Autodesk Inventor part; units mm, degrees
ref_plane "Work Plane1" through (0, 2.2914, -3.9688) normal (0, 0.8660254, 0.5) x (-1, 0, 0)
ref_plane "Work Plane2: Hex Center" through (-3.4449, 0, 0) normal (1, 0, 0) x (0, 0, -1)
ref_plane "YZ Plane" through (0, 0, 0) normal (1, 0, 0) x (0, 1, 0)
sketch "Sketch1: Hex" plane through (0, 0, 0) normal (1, 0, 0) x (0, 1, 0)
  line L0 (-2.2914, 3.9688) -> (2.2914, 3.9687)
  line L1 (2.2914, 3.9687) -> (4.5827, 0)
  line L2 (4.5827, 0) -> (2.2914, -3.9688)
  line L3 (2.2914, -3.9688) -> (-2.2914, -3.9688)
  line L4 (-2.2914, -3.9688) -> (-4.5827, 0)
  line L5 (-4.5827, 0) -> (-2.2914, 3.9688)
  circle A0 centre (0, 0) radius 0.87
  point P0 (0, 3.9687)
  point P1 (0, -3.9688)
  dimension "hex_angle" = 120
  dimension "hex_size" = 7.9375
  dimension "d1" = 1.7399
extrude "Ex: Hex" add sketch "Sketch1: Hex" against normal blind 6.8898 contours L0 L1 L2 L3 L4 L5 | A0
hole "Hole: Tap" [suppressed]
hole "Hole: Thread" at (0, 0, 0) direction (-1, 0, 0) diameter 3.683 depth 5.842
sketch "Sketch2: Top" plane through (-6.8898, 0, 0) normal (1, 0, 0) x (0, 1, 0)
  circle A0 centre (0, 0) radius 3.9687
  circle A1 centre (0, 0) radius 3.7147
  dimension "d4" = 7.9375
  dimension "d5" = 7.4295
extrude "Ex: Top" add sketch "Sketch2: Top" against normal blind 0.9843 contours A0 | A1
hole "Hole: Tubing" at (0, 0, 0) direction (-1, 0, 0) diameter 1.7399 end through all
chamfer "Chamfer1: Top (side)" distance 0.254 angle 45 1 edges at (-7.874, -3.9687, 0)
chamfer "Chamfer2: Top (hole)" distance 0.254 angle 45 1 edges at (-7.874, 0, 0.87)
sketch "Sketch3: Reference: Nut Chamfer" plane through (0, 0, 0) normal (1, 0, 0) x (0, 0, -1)
  circle A0 centre (0, 0) radius 3.9688
  line L0 (3.9688, 2.2914) -> (0, 4.5827)
ref_plane "Work Plane1" through (0, 2.2914, -3.9688) normal (0, 0.8660254, 0.5) x (-1, 0, 0)
sketch "Sketch4: Chamfer (nut)" plane through (0, 0, 0) normal (0, 0.8660254, 0.5) x (-1, 0, 0)
  line L0 (0, -3.9688) -> (0, -4.5827)
  line L1 (0, -4.5827) -> (0.3545, -4.5827)
  line L2 (0.3545, -4.5827) -> (0, -3.9688)
  line L3 (0, 3.9688) -> (0, -3.9688)
  line L4 (8.2677, 0) -> (-1.378, 0)
  line L5 (0, -4.5827) -> (6.8898, -4.5827)
  point P0 (0, 0)
  dimension "chamfer_angle" = 30
revolve "Revolution: Chamfer (nut)" cut sketch "Sketch4: Chamfer (nut)" angle 360 about axis through (-10, 0, 0) along (1, 0, 0)
ref_plane "Work Plane2: Hex Center" through (-3.4449, 0, 0) normal (1, 0, 0) x (0, 0, -1)
mirror "Mirror: Chamfer (nut)" about plane through (-3.4449, 0, 0) normal (1, 0, 0) of "Revolution: Chamfer (nut)"
properties part number "Nut for Precision Compression Fitting"
Geometry check sheet. Reference: the model listing, model coordinates, mm. Round coordinates to 2 decimals unless told otherwise and drop trailing zeros. Loops run counter-clockwise (first coordinate to the right, second up) from the corner with the lowest first, then second, coordinate; pieces in that order, holes last. Notation, with made-up numbers: M 84.25,68 L 135.25,68 A19 cw 135.25,73 Z; hole C 5.5,36 d11. An arc over 180 degrees is marked long. Return JSON: item names as keys, results as strings. Group by question number.
(1) Section check A-A, the plane x = -5.25. Enter the section's corners in (y, z), and give its area (3 significant figures).
(2) Section check B-B, the plane x = -6.25. Enter the section's corners in (y, z), and give its area (3 significant figures).
(3) Scan lines: line 1 along Z through (x, y) = (-2.5, 0); line 2 along Z through (x, y) = (-7.1, 0). Record each from-to range of solid material in increasing order. Write a range as [from, to].
(4) Mould release check, pull along Z, two halves, no side actions. Record for faces 1 (the face through (0, 1, -2)), 2 (the face through (-2.962, 1.634, -0.85)), 3 (the face through (-6.78, 2.09, 3.6)), 4 (the face through (-0.086, 4.118, 0.01)): pulls with the +Z half, pulls with the -Z half, needs draft (parallel to the pull), parting line crosses it, or undercut.
(5) Go/stop test with a flat-tipped pin: pin 1 (1.1 mm diameter, centred on y = 0, z = 0.5, fed in from +X). Record where the tip stops, or that it passes through.
Data:
{
 "1": {"outline": "M -4.58,0 L -2.29,-3.97 L 2.29,-3.97 L 4.58,0 L 2.29,3.97 L -2.29,3.97 Z; hole C 0,0 d3.68", "area": "43.9 mm²"},
 "2": {"outline": "M -4.58,0 L -2.29,-3.97 L 2.29,-3.97 L 4.58,0 L 2.29,3.97 L -2.29,3.97 Z; hole C 0,0 d1.74", "area": "52.2 mm²"},
 "3": {"line 1": "[-3.97, -1.84], [1.84, 3.97]", "line 2": "[-3.97, -0.87], [0.87, 3.97]"},
 "4": {"face 1": "needs draft", "face 2": "undercut", "face 3": "pulls with the +Z half", "face 4": "parting line crosses it"},
 "5": {"pin 1": "x = -5.84"}
}
